from build123d import *

# Parameters (mm, degrees)
BOSS_EXTRUDE1_DEPTH = 12
BOSS_EXTRUDE2_DEPTH = 2
BOSS_EXTRUDE3_DEPTH = 3
SKETCH4_W           = 10
SKETCH4_H           = 2
CUT_EXTRUDE1_DEPTH  = 6
SKETCH5_W           = 10
SKETCH5_H           = 2
CUT_EXTRUDE2_DEPTH  = 6
SKETCH6_W           = 10
SKETCH6_H           = 2
CUT_EXTRUDE3_DEPTH  = 6


with BuildPart() as part:
    # Sketch1 → Boss-Extrude1 (new body)
    with BuildSketch(Plane(origin=(0, 0, 0), x_dir=(1, 0, 0), z_dir=(0, 1, 0))):
        Polygon((109.556624327, -4.42820323), (-109.556624327, -4.42820323), (-112.113248654, 0), (-2.55662435, 189.757639654), (2.556624303, 189.757639654), (112.113248654, 0), align=None)
        Polygon((-107.82457352, -1.42820323), (-108.649147039, 0), (-99.473720558, 15.892304845), (-89.473720559, -1.42820323), align=None, mode=Mode.SUBTRACT)
        Polygon((-0.824573543, 186.757639627), (0.824573481, 186.757639627), (9.999999979, 170.86533478), (-10.000000021, 170.86533478), align=None, mode=Mode.SUBTRACT)
        Polygon((108.649147039, 0), (107.82457353, -1.428203222), (89.473720569, -1.428203222), (99.473720569, 15.892304853), align=None, mode=Mode.SUBTRACT)
        Polygon((-11.732050803, 167.865334802), (11.732050803, 167.865334802), (97.741669765, 18.89230486), (86.00961895, -1.428203229), (-86.009618944, -1.428203229), (-97.741669751, 18.892304845), align=None, mode=Mode.SUBTRACT)
    extrude(amount=BOSS_EXTRUDE1_DEPTH)

    # Sketch1<4> → Boss-Extrude2 (add)
    with BuildSketch(Plane(origin=(0, 0, 0), x_dir=(1, 0, 0), z_dir=(0, 1, 0))):
        Polygon((11.732050803, 167.865334802), (-11.732050803, 167.865334802), (-97.741669751, 18.892304845), (-86.009618944, -1.428203229), (86.00961895, -1.428203229), (97.741669765, 18.89230486), align=None)
        with BuildLine():
            Line((-85.566243251, 2.803847594), (-93.854918378, 17.160254041))
            ThreePointArc((-93.854918378, 17.160254041), (-82.532377591, 14.126388381), (-85.566243251, 2.803847594))
        make_face(mode=Mode.SUBTRACT)
        Polygon((-1e-08, 9.732050841), (4.99999999, 1.071796803), (-5.00000001, 1.071796803), align=None, mode=Mode.SUBTRACT)
        Polygon((-45.071796745, 87.798692801), (-55.071796745, 87.798692801), (-50.071796745, 96.458946839), align=None, mode=Mode.SUBTRACT)
        Polygon((82.210580848, 14.312177834), (92.210580848, 14.312177834), (87.210580848, 5.651923796), align=None, mode=Mode.SUBTRACT)
        with BuildLine():
            Line((48.91709624, 98.458946834), (41.607695163, 85.798692796))
            Line((41.607695163, 85.798692796), (56.226497316, 85.798692796))
            Line((56.226497316, 85.798692796), (94.854918412, 18.892304841))
            Line((94.854918412, 18.892304841), (93.36528139, 16.312177834))
            Line((93.36528139, 16.312177834), (78.746479233, 16.312177834))
            Line((78.746479233, 16.312177834), (86.055880312, 3.651923793))
            Line((86.055880312, 3.651923793), (84.566243293, 1.071796793))
            Line((84.566243293, 1.071796793), (7.309401088, 1.071796793))
            Line((7.309401088, 1.071796793), (2e-09, 13.732050847))
            Line((2e-09, 13.732050847), (-7.309401077, 1.071796786))
            Line((-7.309401077, 1.071796786), (-84.566243251, 1.071796786))
            ThreePointArc((-84.566243251, 1.071796786), (-80.800326783, 15.126388381), (-94.854918378, 18.892304849))
            Line((-94.854918378, 18.892304849), (-56.226497283, 85.798692801))
            Line((-56.226497283, 85.798692801), (-41.60769513, 85.798692801))
            Line((-41.60769513, 85.798692801), (-48.917096207, 98.458946839))
            Line((-48.917096207, 98.458946839), (-10.288675112, 165.365334792))
            Line((-10.288675112, 165.365334792), (-7.309401077, 165.365334792))
            Line((-7.309401077, 165.365334792), (0, 152.705080754))
            Line((0, 152.705080754), (7.309401077, 165.365334792))
            Line((7.309401077, 165.365334792), (10.288675142, 165.365334792))
            Line((10.288675142, 165.365334792), (48.91709624, 98.458946834))
        make_face(mode=Mode.SUBTRACT)
        Polygon((45.071796778, 87.798692803), (50.071796778, 96.458946841), (55.071796778, 87.798692803), align=None, mode=Mode.SUBTRACT)
        Polygon((0, 156.705080761), (-5, 165.365334799), (5, 165.365334799), align=None, mode=Mode.SUBTRACT)
    extrude(amount=BOSS_EXTRUDE2_DEPTH)

    # Sketch2 → Boss-Extrude3 (add)
    with BuildSketch(Plane.XZ):
        Polygon((101.205771363, -18.892304847), (87.741669751, 4.42820323), (-87.741669751, 4.42820323), (-101.205771368, -18.892304847), (-13.464101652, -170.86533478), (13.464101609, -170.86533478), align=None)
        Polygon((-11.732050819, -167.865334802), (11.732050795, -167.865334802), (97.741669739, -18.892304852), (86.009618931, 1.42820323), (-86.009618931, 1.42820323), (-97.741669763, -18.892304852), align=None, mode=Mode.SUBTRACT)
    extrude(amount=BOSS_EXTRUDE3_DEPTH)

    # Sketch4 → Cut-Extrude1 (cut)
    with BuildSketch(Plane.XY.offset(4.42820323)):
        with Locations((-79.741669751, -1)):
            Rectangle(SKETCH4_W, SKETCH4_H)
    extrude(amount=-CUT_EXTRUDE1_DEPTH, mode=Mode.SUBTRACT)

    # Sketch5 → Cut-Extrude2 (cut)
    with BuildSketch(Plane(origin=(-84.084936503, 0, -48.546460711), x_dir=(-0.4999999998935114, 0, 0.86602540384592), z_dir=(-0.86602540384592, 0, -0.4999999998935114))):
        with Locations((26.241669739, -1)):
            Rectangle(SKETCH5_W, SKETCH5_H)
    extrude(amount=-CUT_EXTRUDE2_DEPTH, mode=Mode.SUBTRACT)

    # Sketch6 → Cut-Extrude3 (cut)
    with BuildSketch(Plane(origin=(84.084936484, 0, -48.546460721), x_dir=(-0.5000000000540236, 0, -0.8660254037532481), z_dir=(0.8660254037532481, 0, -0.5000000000540236))):
        with Locations((53.499999991, -1)):
            Rectangle(SKETCH6_W, SKETCH6_H)
    extrude(amount=-CUT_EXTRUDE3_DEPTH, mode=Mode.SUBTRACT)


solid = part.part
Can you work these out from the model? Positions are in its coordinate system, mm. A direction names the side the tool comes from. Round coordinates to 2 decimals unless told otherwise and drop trailing zeros. Order: outer loops, then holes, each group sorted by start corner. A loop starts at its lowest first (then second) coordinate and runs counter-clockwise, first axis right, second up. Notation, with made-up numbers: M 28,-21.75 L 78,-21.75 A14 cw 78,5.25 Z; hole C 31,-20.75 d7. An arc over 180 degrees is marked long. Use a Markdown table: item, result.
1) If we mould it in two halves opening along X, with no side actions, what happens to faces 1 (the face through (-89.65, 0.99, -9.88)), 2 (the face through (0, 6, -189.758))? For each: +X half, -X half, draft (parallel to the pull), parting line (faces both ways), or undercut.
Geometry says:
| item | result |
|---|---|
| face 1 | undercut |
| face 2 | draft |
2) Imagine slicing it at A-A (z = -79). List the corners of the cut face in (x, y) for me.
Geometry says:
| item | result |
|---|---|
| outline | M -66.5,-3 L -63.04,-3 L -63.04,0 L -60.15,0 L -60.15,2 L -63.04,2 L -63.04,12 L -66.5,12 Z; M 60.15,0 L 63.04,0 L 63.04,-3 L 66.5,-3 L 66.5,12 L 63.04,12 L 63.04,2 L 60.15,2 Z |
3) I'm going to push flat-ended pins straight in: P1, Ø1.5, axis at y = 2, z = -161, coming from the +X side; P2, Ø8, axis at x = -32, y = -1.5, coming from the -Z side; P3, Ø7, axis at x = -104.5, z = -8, coming from the -Y side. Where does each tip first touch, or does it pass through?
Geometry says:
| item | result |
|---|---|
| P1 | stops at x = 19.59 |
| P2 | stops at z = -145.69 |
| P3 | stops at y = 0 |
4) On a 3-axis mill with a long thin cutter (end or side, diameter ignored), from which of +Z, -Z, +X, -X, +Y, -Y can I reach the whole of each face in a straight line? I mean faces 3 (the face through (54.135, 6.93, -94.422)), 4 (the face through (91.958, -1.479, -8.874)), 5 (the face through (45.314, 0.986, -92.217)). Say none if no direction works.
Geometry says:
| item | result |
|---|---|
| face 3 | +Y |
| face 4 | -Y |
| face 5 | +Y, -Y |
5) Imagine slicing it at C-C (x = -63). List the corners of the cut face in (y, z) for me.
Geometry says:
| item | result |
|---|---|
| outline | M -3,-85.07 L 12,-85.07 L 12,-79.07 L 2,-79.07 L 2,-74.07 L 0,-74.07 L 0,-79.07 L -3,-79.07 Z; M -3,1.43 L 0,1.43 L 0,-1.07 L 2,-1.07 L 2,1.43 L 12,1.43 L 12,4.43 L -3,4.43 Z |
6) Imagine slicing it at B-B (y = 9.25). List the corners of the cut face in (x, z) for me, then the cut area to 3 significant figures.
Geometry says:
| item | result |
|---|---|
| outline | M -112.11,0 L -2.56,-189.76 L 2.56,-189.76 L 112.11,0 L 109.56,4.43 L -109.56,4.43 Z; hole M -108.65,0 L -99.47,-15.89 L -89.47,1.43 L -107.82,1.43 Z; hole M -97.74,-18.89 L -11.73,-167.87 L 11.73,-167.87 L 97.74,-18.89 L 86.01,1.43 L -86.01,1.43 Z; hole M -10,-170.87 L -0.82,-186.76 L 0.82,-186.76 L 10,-170.87 Z; hole M 89.47,1.43 L 99.47,-15.89 L 108.65,0 L 107.82,1.43 Z |
| area | 2,180 mm² |
7) Imagine slicing it at D-D (z = -161). List the corners of the cut face in (x, y) for me, then the cut area to 3 significant figures.
Geometry says:
| item | result |
|---|---|
| outline | M -19.16,-3 L -15.7,-3 L -15.7,0 L -12.81,0 L -12.81,2 L -15.7,2 L -15.7,12 L -19.16,12 Z; M -4.79,0 L -2.48,0 L -2.48,2 L -4.79,2 Z; M 2.48,0 L 4.79,0 L 4.79,2 L 2.48,2 Z; M 12.81,0 L 15.7,0 L 15.7,-3 L 19.16,-3 L 19.16,12 L 15.7,12 L 15.7,2 L 12.81,2 Z |
| area | 125 mm² |
8) If I drill on line 1 along X through (y, z) = (3.25, -151); line 2 along X through (y, z) = (3.25, -68); line 3 along Z through (x, y) = (49, 10), over which ranges is the centre line in solid material (lowest first)?
Geometry says:
| item | result |
|---|---|
| line 1 | x = -24.93 to -21.47, 21.47 to 24.93 |
| line 2 | x = -72.85 to -69.39, 69.39 to 72.85 |
| line 3 | z = -109.32 to -103.32, 1.43 to 4.43 |
